```python
from build123d import *

# Parameters (mm, degrees)
SKETCH1_R                = 100
BOSS_EXTRUDE1_DEPTH      = 3.175
FILLET1_R                = 3
CIRPATTERN1_COUNT        = 2
FILLET1_OF_CIRPATTERN1_R = 3
SKETCH2_R                = 2.65
CUT_EXTRUDE1_DEPTH       = 174.229104079
CIRPATTERN2_COUNT        = 8


with BuildPart() as part:
    # Sketch1 → Boss-Extrude1 (new, symmetric)
    with BuildSketch(Plane(origin=(0, 0, 0), x_dir=(1, 0, 0), z_dir=(0, 1, 0))):
        with BuildLine():
            Line((-111.986312116, 1.750970805), (-132, 0))
            ThreePointArc((-132, 0), (-115.815804966, -46.398149165), (-79.477414809, -79.477414809))
            ThreePointArc((-79.477414809, -79.477414809), (-78.32708198, -80.19539315), (-77.284459499, -81.062397694))
            ThreePointArc((-77.284459499, -81.062397694), (103.297481806, 43.285450818), (-111.986312116, 1.750970805))
        make_face()
        with Locations(Location((0, 0, 0), (0, 0, 270))):
            Circle(SKETCH1_R, mode=Mode.SUBTRACT)
    boss_extrude1 = extrude(amount=BOSS_EXTRUDE1_DEPTH, both=True)

    # Fillet1
    fillet1_edges = [part.edges().sort_by_distance(p)[0] for p in [
        (-111.986312116, 0, -1.750970805),
    ]]
    fillet(fillet1_edges, radius=FILLET1_R)

    # CirPattern1: Boss-Extrude1 ×2 about axis
    cirpattern1_axis = Axis((0, 0, 0), (0, 1, 0))
    for i in range(1, CIRPATTERN1_COUNT):
        add(boss_extrude1.rotate(cirpattern1_axis, i * 360 / CIRPATTERN1_COUNT))

    # Fillet1 of CirPattern1
    fillet1_of_cirpattern1_edges = [part.edges().sort_by_distance(p)[0] for p in [
        (111.986312116, 0, 1.750970805),
    ]]
    fillet(fillet1_of_cirpattern1_edges, radius=FILLET1_OF_CIRPATTERN1_R)

    # Sketch2 → Cut-Extrude1 (cut, through all)
    with BuildSketch(Plane(origin=(0, 3.175, 0), x_dir=(1, 0, 0), z_dir=(0, 1, 0))):
        with Locations(Location((-102.388137587, -27.434818781, 0), (0, 0, 270))):
            Circle(SKETCH2_R)
    cut_extrude1 = extrude(amount=-CUT_EXTRUDE1_DEPTH, mode=Mode.SUBTRACT)

    # CirPattern2: Cut-Extrude1 ×8 about axis
    cirpattern2_axis = Axis((0, 0, 0), (0, 1, 0))
    for i in range(1, CIRPATTERN2_COUNT):
        add(cut_extrude1.rotate(cirpattern2_axis, i * 360 / CIRPATTERN2_COUNT), mode=Mode.SUBTRACT)


solid = part.part
```
Geometry check sheet. Reference: the model listing, model coordinates, mm. Round coordinates to 2 decimals unless told otherwise and drop trailing zeros. Order: outer loops, then holes, each group sorted by start corner. A loop starts at its lowest first (then second) coordinate and runs counter-clockwise, first axis right, second up. Notation, with made-up numbers: M -21,-17.5 L 34,-17.5 A31 cw 34,6.5 Z; hole C 48.25,24 d6. An arc over 180 degrees is marked long. Answer as CSV lines item,"result".
1) Sectioned sample at A-A on z = -11. Record the cut outline in (x, y) (3 decimals), and give its area (3 significant figures).
Entries:
outline,"M -111.459,-3.175 L -99.393,-3.175 L -99.393,3.175 L -111.459,3.175 Z; M 99.393,-3.175 L 130.417,-3.175 L 130.417,3.175 L 99.393,3.175 Z"
area,"274 mm2"
2) Thickness scan on probe 1 along Z at (x, y) = (-52, -2); probe 2 along Z at (x, y) = (91, 2.5); probe 3 along Z at (x, y) = (74.5, -1.25). Record the ranges inside material, lowest first. Write a range as [from, to].
Entries:
probe 1,"[-99.2, -85.42], [85.42, 89.34], [94.25, 99.2]"
probe 2,"[-72.28, -41.46], [41.46, 50.47], [55.53, 65.29]"
probe 3,"[-83.63, -66.71], [66.71, 83.63]"
3) Gauge pin test, flat ends, axial feed: pin 1 Ø1 at (y, z) = (0.5, -55.5) entering from -X; pin 2 Ø1 at (x, y) = (-30.5, -2.5) entering from +Z. Record the tip position at first contact, or that the pin passes through.
Entries:
pin 1,"x = -97.57"
pin 2,"z = 107.91"
4) Mould release check, pull along X, two halves, no side actions. Record for faces 1 (the face through (-116.197, 0.044, 45.817)), 2 (the face through (94.25, 0.04, 51.99)), 3 (the face through (40.394, 0.044, 104.462)): +X half, -X half, draft (parallel to the pull), parting line (faces both ways), or undercut.
Entries:
face 1,"-X half"
face 2,"undercut"
face 3,"parting line"
5) Sectioned sample at C-C on y = -0.5. Give the number of separate pieces and of enclosed holes in the cut face, and give its area (3 significant figures).
Entries:
separate pieces,"1"
enclosed holes,"9"
area,"10,000 mm2"
6) Sectioned sample at B-B on x = 0. Record the cut outline in (y, z) (3 decimals).
Entries:
outline,"M -3.175,-112 L 3.175,-112 L 3.175,-100 L -3.175,-100 Z; M -3.175,100 L 3.175,100 L 3.175,112 L -3.175,112 Z"
